```python
from build123d import *

# Parameters (mm, degrees)
SKETCH_3_W      = 60
SKETCH_3_H      = 10
EXTRUDE_1_DEPTH = 10
SKETCH_4_W      = 60
SKETCH_4_H      = 10
EXTRUDE_2_DEPTH = 5
SKETCH_5_W      = 60
SKETCH_5_H      = 5
EXTRUDE_3_DEPTH = 5
SKETCH_6_W      = 60
SKETCH_6_H      = 7.5
EXTRUDE_4_DEPTH = 10


with BuildPart() as part:
    # 草图3 → 凸台-拉伸1 (new body)
    with BuildSketch(Plane.XZ.offset(-0.087836635)):
        with Locations((26.631510997, 9.323973154)):
            Rectangle(SKETCH_3_W, SKETCH_3_H)
    extrude(amount=EXTRUDE_1_DEPTH)

    # 草图4 → 凸台-拉伸2 (add)
    with BuildSketch(Plane.XY.offset(14.323973154)):
        with Locations((26.631510997, -4.912163365)):
            Rectangle(SKETCH_4_W, SKETCH_4_H)
    extrude(amount=EXTRUDE_2_DEPTH)

    # 草图5 → 凸台-拉伸3 (add)
    with BuildSketch(Plane(origin=(0, 0.087836635, 0), x_dir=(1, 0, 0), z_dir=(0, 1, 0))):
        with Locations((26.631510997, -16.823973154)):
            Rectangle(SKETCH_5_W, SKETCH_5_H)
    extrude(amount=EXTRUDE_3_DEPTH)

    # 草图6 → 凸台-拉伸4 (add)
    with BuildSketch(Plane.XY.offset(19.323973154)):
        with Locations((26.631510997, 1.337836635)):
            Rectangle(SKETCH_6_W, SKETCH_6_H)
    extrude(amount=EXTRUDE_4_DEPTH)


solid = part.part
```
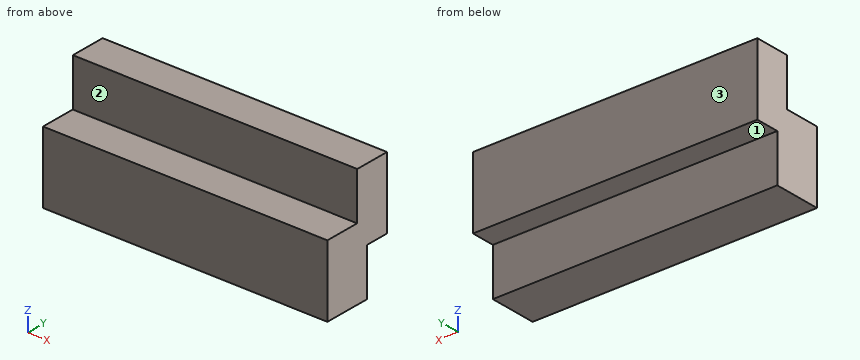
Build history of the part. All positions in model axes, mm. Face numbers are marked on the shaded views. A direction names the side the tool comes from. Coordinates: 2 decimals unless noted, no trailing zeros. Order: outer loops, then holes, each group sorted by start corner. A loop starts at its lowest first (then second) coordinate and runs counter-clockwise, first axis right, second up. Notation, with made-up numbers: M -21,-23.5 L 8,-23.5 A22 cw 8,-13.5 Z; hole C 37.25,-20 d7. An arc over 180 degrees is marked long. One line per question, with ' | ' between items. Start each with the question number.
1. Cut at B-B (z = 10.75). Write the cut outline in (x, y), plus the area to 3 significant figures.
2. Cut at C-C (y = 3.75). Write the cut outline in (x, z), plus the area to 3 significant figures.
3. Flat gauge pins, fed straight in: P1, Ø5, axis at x = 30, z = 23, coming from the -Y side; P2, Ø2, axis at x = 13.5, y = -7.5, coming from the +Z side; P3, Ø3, axis at x = 20.5, z = 7.5, coming from the +Y side. Where does each tip first touch, or does it go through?
4. Wall check: line 1 along Z through (x, y) = (36, 0.5); line 2 along Y through (x, z) = (38.5, 20); line 3 along Z through (x, y) = (43.5, -3). Give the ranges that are in metal, low to high. Write a range as [from, to].
5. Tool access for the marked faces 1, 2 and 3: list every direction of +Z, -Z, +X, -X, +Y, -Y with a clear straight run to the whole face (end or side of a thin tool).
6. Cut at A-A (x = 8). Write the cut outline in (y, z), plus the area to 3 significant figures.
The answers:
1) outline: M -3.37,-9.91 L 56.63,-9.91 L 56.63,0.09 L -3.37,0.09 Z | area: 600 mm2
2) outline: M -3.37,14.32 L 56.63,14.32 L 56.63,29.32 L -3.37,29.32 Z | area: 900 mm2
3) P1: stops at y = -2.41 | P2: stops at z = 19.32 | P3: stops at y = 0.09
4) line 1: z = [14.32, 29.32] | line 2: y = [-2.41, 5.09] | line 3: z = [4.32, 19.32]
5) face 1: -Z, +X, -X, +Y | face 2: +Z, +X, -X, -Y | face 3: +Z, -Z, +X, -X, +Y
6) outline: M -9.91,4.32 L 0.09,4.32 L 0.09,14.32 L 5.09,14.32 L 5.09,29.32 L -2.41,29.32 L -2.41,19.32 L -9.91,19.32 Z | area: 250 mm2
